from build123d import *

# Parameters (mm, degrees)
SKETCH1_R           = 92.5
BOSS_EXTRUDE1_DEPTH = 13
SKETCH2_R           = 17.5
CUT_EXTRUDE1_DEPTH  = 132.459119121
SKETCH3_R           = 10
CUT_EXTRUDE2_DEPTH  = 10.618282
CIRPATTERN1_START   = 2.381718456
CIRPATTERN1_DEPTH   = 10.618281544


# Read off the part's stored shape, not the designer's step: CirPattern1
with BuildPart() as part:
    # Sketch1 → Boss-Extrude1 (new body)
    with BuildSketch(Plane(origin=(0, 0, 0), x_dir=(1, 0, 0), z_dir=(0, 1, 0))):
        with Locations(Location((0, 0, 0), (0, 0, 90))):
            Circle(SKETCH1_R)
    extrude(amount=BOSS_EXTRUDE1_DEPTH)

    # Sketch2 → Cut-Extrude1 (cut, through all)
    with BuildSketch(Plane(origin=(0, 0, 0), x_dir=(1, 0, 0), z_dir=(0, 1, 0))):
        with Locations(Location((0, 0, 0), (0, 0, 90))):
            Circle(SKETCH2_R)
    extrude(amount=CUT_EXTRUDE1_DEPTH, mode=Mode.SUBTRACT)

    # Sketch3 → Cut-Extrude2 (cut)
    with BuildSketch(Plane(origin=(0, 13, 0), x_dir=(1, 0, 0), z_dir=(0, 1, 0))):
        with Locations((-16.735268537, 0)):
            Circle(SKETCH3_R)
    extrude(amount=-CUT_EXTRUDE2_DEPTH, mode=Mode.SUBTRACT)

    # CirPattern1 outline → CirPattern1 (cut)
    with BuildSketch(Plane(origin=(0, 0, 0), x_dir=(1, 0, 0), z_dir=(0, 1, 0)).offset(CIRPATTERN1_START)):
        with BuildLine():
            ThreePointArc((-13.766320154, 10.804555956), (-5.407797402, 16.643489035), (4.786428306, 16.83270935))
            ThreePointArc((4.786428306, 16.83270935), (-8.261652327, 25.426751357), (-13.766320154, 10.804555956))
        make_face()
        with BuildLine():
            ThreePointArc((17.487945603, 0.64942942), (21.629286596, 15.714596562), (6.02171647, 16.431339895))
            ThreePointArc((6.02171647, 16.431339895), (14.157797402, 10.286241915), (17.487945603, 0.64942942))
        make_face()
        with BuildLine():
            ThreePointArc((4.786428306, -16.83270935), (-5.407797402, -16.643489035), (-13.766320154, -10.804555956))
            ThreePointArc((-13.766320154, -10.804555956), (-8.261652327, -25.426751357), (4.786428306, -16.83270935))
        make_face()
        with BuildLine():
            ThreePointArc((17.487945603, -0.64942942), (14.157797402, -10.286241915), (6.02171647, -16.431339895))
            ThreePointArc((6.02171647, -16.431339895), (21.629286596, -15.714596562), (17.487945603, -0.64942942))
        make_face()
    extrude(amount=CIRPATTERN1_DEPTH, mode=Mode.SUBTRACT)


solid = part.part
Model file for the job. Use its own axes, mm. A direction names the side the tool comes from. Round coordinates to 2 decimals unless told otherwise and drop trailing zeros. Loops run counter-clockwise (first coordinate to the right, second up) from the corner with the lowest first, then second, coordinate; pieces in that order, holes last. Notation, with made-up numbers: M 69,70 L 98,70 A26 ccw 98,91 Z; hole C -7,63.25 d6. An arc over 180 degrees is marked long. One line per question, with ' | ' between items.
1) Drill centre lines: line 1 along X through (y, z) = (9, -5); line 2 along Z through (x, y) = (3, 1); line 3 along Z through (x, y) = (14.5, 8.5). Where is each one in solid material? Low to high.
Solved:
line 1: x = -92.36 to -25.4, 22.29 to 92.36 | line 2: z = -92.45 to -17.24, 17.24 to 92.45 | line 3: z = -91.36 to -19.79, 19.79 to 91.36
2) Band-saw the part on A-A (x = 0). Give the cut face in (y, z), then the cut area to 3 significant figures.
Solved:
outline: M 0,-92.5 L 13,-92.5 L 13,-24.48 L 2.38,-24.48 L 2.38,-17.5 L 0,-17.5 Z; M 0,17.5 L 2.38,17.5 L 2.38,24.48 L 13,24.48 L 13,92.5 L 0,92.5 Z | area: 1,800 mm²
3) Mould opens along X. For faces 3 (the flat face through (17, 2.382, 12)), 4 (the flat face through (19, 13, 1)), 5 (the cylindrical face through (90.3, 6.41, 20.05)) say: +X half, -X half, draft (parallel to the pull), parting line (faces both ways), or undercut.
Solved:
face 3: undercut | face 4: draft | face 5: parting line
4) Band-saw the part on D-D (x = -81). Give the cut face in (y, z).
Solved:
outline: M 0,-44.67 L 13,-44.67 L 13,44.67 L 0,44.67 Z
5) 3-axis set-ups, long thin cutter, end or side, ignore diameter. For faces 1 (the cylindrical face through (21.774, 7.617, -15.51)), 2 (the flat face through (19, 0, 1)): which of +Z, -Z, +X, -X, +Y, -Y reach the whole face in a straight line?
Solved:
face 1: +Y | face 2: +Z, -Z, +X, -X, -Y
6) Band-saw the part on C-C (z = 58). Give the cut face in (x, y), then the cut area to 3 significant figures.
Solved:
outline: M -72.06,0 L 72.06,0 L 72.06,13 L -72.06,13 Z | area: 1,870 mm²
7) Flat gauge pins, fed straight in: pin 1 (5.5 mm diameter, centred on x = 10.5, z = 7, fed in from +Y); pin 2 (4.5 mm diameter, centred on x = -7, z = -16, fed in from +Y); pin 3 (4 mm diameter, centred on y = 2.5, z = 50, fed in from +X); pin 4 (5 mm diameter, centred on y = 5, z = 46.5, fed in from +X). Where does each tip first touch, or does it go through?
Solved:
pin 1: passes through | pin 2: stops at y = 2.38 | pin 3: stops at x = 79.07 | pin 4: stops at x = 81.36
8) Band-saw the part on B-B (y = 9). Give the cut face in (x, z), then the cut area to 3 significant figures.
Solved:
outline: C 0,0 d185; hole M -14.53,-9.75 A17.5 ccw -13.77,-10.8 A10 ccw long 4.79,-16.83 A17.5 ccw 6.02,-16.43 A10 ccw long 17.49,-0.65 A17.5 ccw 17.49,0.65 A10 ccw long 6.02,16.43 A17.5 ccw 4.79,16.83 A10 ccw long -13.77,10.8 A17.5 ccw -14.53,9.75 A10 ccw long Z | area: 25,100 mm²
